from build123d import *

# Parameters (mm, degrees)
F1_W          = 80
F1_H          = 40
F2_DEPTH      = 250
F3_R          = 4
F3_R_2        = 3.4
F4_DEPTH      = 250.001
F4_DEPTH_BACK = 250.001
F6_DEPTH      = 250.001
F6_DEPTH_BACK = 250.001
F8_DEPTH      = 250.001
F8_DEPTH_BACK = 250.001
F9_R          = 1


with BuildPart() as f2:
    # F1 (on Front) → F2 (new body, symmetric)
    with BuildSketch(Plane.XZ):
        Rectangle(F1_W, F1_H)
    extrude(amount=F2_DEPTH, both=True)

    # F3 (on Front) → F4 (cut, two sides)
    with BuildSketch(Plane.XZ) as f4_sk:
        with Locations((-33.5, 13.5)):
            Circle(F3_R)
        with Locations((-33.5, -13.5)):
            Circle(F3_R)
        with Locations((33.5, -13.5)):
            Circle(F3_R)
        with Locations((33.5, 13.5)):
            Circle(F3_R)
        with Locations((-20, 0)):
            Circle(F3_R_2)
        with Locations((20, 0)):
            Circle(F3_R_2)
    extrude(amount=-F4_DEPTH, mode=Mode.SUBTRACT)
    extrude(f4_sk.sketch, amount=F4_DEPTH_BACK, mode=Mode.SUBTRACT)

    # F5 (on Front) → F6 (cut, two sides)
    with BuildSketch(Plane.XZ) as f6_sk:
        with BuildLine():
            Line((-15.8, 20), (-24.2, 20))
            Line((-24.2, 20), (-24.2, 16))
            Line((-24.2, 16), (-27.25, 16))
            Line((-27.25, 16), (-27.25, 8.8609854211))
            ThreePointArc((-27.25, 8.8609854211), (-20, 5.5), (-12.75, 8.8609854211))
            Line((-12.75, 8.8609854211), (-12.75, 16))
            Line((-12.75, 16), (-15.8, 16))
            Line((-15.8, 16), (-15.8, 20))
        make_face()
        with BuildLine():
            Line((-40, 4.2), (-40, -4.2))
            Line((-40, -4.2), (-36, -4.2))
            Line((-36, -4.2), (-36, -7.25))
            Line((-36, -7.25), (-28.8609854211, -7.25))
            ThreePointArc((-28.8609854211, -7.25), (-25.5, 0), (-28.8609854211, 7.25))
            Line((-28.8609854211, 7.25), (-36, 7.25))
            Line((-36, 7.25), (-36, 4.2))
            Line((-36, 4.2), (-40, 4.2))
        make_face()
        with BuildLine():
            Line((-24.2, -20), (-15.8, -20))
            Line((-15.8, -20), (-15.8, -16))
            Line((-15.8, -16), (-12.75, -16))
            Line((-12.75, -16), (-12.75, -8.8609854211))
            ThreePointArc((-12.75, -8.8609854211), (-20, -5.5), (-27.25, -8.8609854211))
            Line((-27.25, -8.8609854211), (-27.25, -16))
            Line((-27.25, -16), (-24.2, -16))
            Line((-24.2, -16), (-24.2, -20))
        make_face()
        with BuildLine():
            ThreePointArc((27.25, -8.8609854211), (20, -5.5), (12.75, -8.8609854211))
            Line((12.75, -8.8609854211), (12.75, -16))
            Line((12.75, -16), (15.8, -16))
            Line((15.8, -16), (15.8, -20))
            Line((15.8, -20), (24.2, -20))
            Line((24.2, -20), (24.2, -16))
            Line((24.2, -16), (27.25, -16))
            Line((27.25, -16), (27.25, -8.8609854211))
        make_face()
        with BuildLine():
            Line((36, -4.2), (40, -4.2))
            Line((40, -4.2), (40, 4.2))
            Line((40, 4.2), (36, 4.2))
            Line((36, 4.2), (36, 7.25))
            Line((36, 7.25), (28.8609854211, 7.25))
            ThreePointArc((28.8609854211, 7.25), (25.5, 0), (28.8609854211, -7.25))
            Line((28.8609854211, -7.25), (36, -7.25))
            Line((36, -7.25), (36, -4.2))
        make_face()
        with BuildLine():
            Line((15.8, 16), (12.75, 16))
            Line((12.75, 16), (12.75, 8.8609854211))
            ThreePointArc((12.75, 8.8609854211), (20, 5.5), (27.25, 8.8609854211))
            Line((27.25, 8.8609854211), (27.25, 16))
            Line((27.25, 16), (24.2, 16))
            Line((24.2, 16), (24.2, 20))
            Line((24.2, 20), (15.8, 20))
            Line((15.8, 20), (15.8, 16))
        make_face()
    extrude(amount=-F6_DEPTH, mode=Mode.SUBTRACT)
    extrude(f6_sk.sketch, amount=F6_DEPTH_BACK, mode=Mode.SUBTRACT)

    # F7 (on Front) → F8 (cut, two sides)
    with BuildSketch(Plane.XZ) as f8_sk:
        with BuildLine():
            Line((6.75, 15), (-6.75, 15))
            ThreePointArc((-6.75, 15), (-8.8713203436, 14.1213203436), (-9.75, 12))
            Line((-9.75, 12), (-9.75, 7.8454559894))
            ThreePointArc((-9.75, 7.8454559894), (-11.6545131981, 5.6939347714), (-14, 4.0341439003))
            Line((-14, 4.0341439003), (-14, -4.0341439003))
            ThreePointArc((-14, -4.0341439003), (-11.6545131981, -5.6939347714), (-9.75, -7.8454559894))
            Line((-9.75, -7.8454559894), (-9.75, -12))
            ThreePointArc((-9.75, -12), (-8.8713203436, -14.1213203436), (-6.75, -15))
            Line((-6.75, -15), (6.75, -15))
            ThreePointArc((6.75, -15), (8.8713203436, -14.1213203436), (9.75, -12))
            Line((9.75, -12), (9.75, -7.8454559894))
            ThreePointArc((9.75, -7.8454559894), (11.6545131981, -5.6939347714), (14, -4.0341439003))
            Line((14, -4.0341439003), (14, 4.0341439003))
            ThreePointArc((14, 4.0341439003), (11.6545131981, 5.6939347714), (9.75, 7.8454559894))
            Line((9.75, 7.8454559894), (9.75, 12))
            ThreePointArc((9.75, 12), (8.8713203436, 14.1213203436), (6.75, 15))
        make_face()
    extrude(amount=-F8_DEPTH, mode=Mode.SUBTRACT)
    extrude(f8_sk.sketch, amount=F8_DEPTH_BACK, mode=Mode.SUBTRACT)

    # F9
    f9_edges = [f2.edges().sort_by_distance(p)[0] for p in [
        (-40, 0, 20),
        (40, 0, 20),
        (40, 0, -20),
        (-40, 0, -20),
    ]]
    fillet(f9_edges, radius=F9_R)


solid = f2.part
The listing builds one solid part. Answer for the finished solid, in the listing's coordinates (mm). A direction names the side the tool comes from. Round coordinates to 2 decimals unless told otherwise and drop trailing zeros. Write each loop counter-clockwise with the first axis right and the second up, starting at its lowest first coordinate (ties: lowest second). Pieces come first, ordered by that corner, then holes. Notation, with made-up numbers: M 3.5,-19 L 39.5,-19 A32 cw 39.5,12 Z; hole C 48.5,35 d8. An arc over 180 degrees is marked long. Write each question's results on one line, items separated by ' | '. Start each with the question number.
Item 1: Which of the six approach directions +Z, -Z, +X, -X, +Y, -Y give full straight-line access (tool end or side, diameter ignored) to faces 1 (the cylindrical face through (20.1, 3.5, -5.5)), 2 (the flat face through (-32, -4, -20))?
Item 2: Find section A-A on x = -1.5. Write down the section's boundary in (y, z).
Item 3: Find section B-B on y = -186.5. Give the number of separate pieces and of enclosed holes in the cut face, and give its area (3 significant figures).
Item 4: Given pin 1 Ø6 at (y, z) = (-45.5, 0.5) entering from -X; pin 2 Ø1 at (x, y) = (-20.5, -186) entering from -Z; pin 3 Ø5.5 at (x, z) = (-20, 0) entering from -Y, each flat-ended and moving along its own axis, determine where each tip first touches the part or whether it passes through.
Item 5: Straight lines are drawn through the part: probe 1 along X at (y, z) = (135, 13); probe 2 along Z at (x, y) = (-33, 104); probe 3 along Z at (x, y) = (20, 75.5). For each, find the intervals that lie inside material, in ascending order.
Item 6: The mould has two halves that part along X. Classify faces 3 (the flat face through (-32, -4, 20)), 4 (the flat face through (40, -4, 11)), 5 (the flat face through (0, -4, -15)): +X half, -X half, draft (parallel to the pull), parting line (faces both ways), or undercut.
Answer block:
1) face 1: +Y, -Y | face 2: -Z, +X, -X, +Y, -Y
2) outline: M -250,-20 L 250,-20 L 250,-15 L -250,-15 Z; M -250,15 L 250,15 L 250,20 L -250,20 Z
3) separate pieces: 1 | enclosed holes: 7 | area: 1,230 mm²
4) pin 1: stops at x = -26.17 | pin 2: stops at z = -5.55 | pin 3: passes through
5) probe 1: x = -40 to -37.47, -29.53 to -27.25, -12.75 to -9.58, 9.58 to 12.75, 27.25 to 29.53, 37.47 to 40 | probe 2: z = -20 to -17.47, -9.53 to -7.25, 7.25 to 9.53, 17.47 to 20 | probe 3: z = -5.5 to -3.4, 3.4 to 5.5
6) face 3: draft | face 4: +X half | face 5: undercut
